Design review of the part built by this model. Coordinates are the model's own, in mm. Coordinates: 2 decimals unless noted, no trailing zeros. Write each loop counter-clockwise with the first axis right and the second up, starting at its lowest first coordinate (ties: lowest second). Pieces come first, ordered by that corner, then holes. Notation, with made-up numbers: (62.5, 66) - (113.5, 66) arc R18 cw to (113.5, 100) - close; hole circle Ø3 at (-29, 30). An arc over 180 degrees is marked (long way). Answer as CSV lines item,"result". Start each with the question number.
Q1. For line 1 along Z through (x, y) = (114.3, 1.85); line 2 along X through (y, z) = (3.7, 139.7); line 3 along X through (y, z) = (2.8, 117), list the stretches that pass through material, from the lowest coordinate up. Write a range as [from, to].
Q2. We need section A-A (z = 139.7). Write out the cut boundary in (x, y), plus the area to 3 significant figures.
Q3. We need section D-D (x = 12.7). Write out the cut boundary in (y, z).
Q4. We need section C-C (z = 38). Write out the cut boundary in (x, y).
Q5. Clearance check with flat-ended pins moving along their axes: pin 1 (2.5 mm diameter, centred on y = 3, z = 118.5, fed in from -X); pin 2 (1.4 mm diameter, centred on x = -6.5, y = 3.5, fed in from +Z). State where each tip first meets the part, or that it passes through.
Q6. We need section B-B (x = 114.3). Write out the cut boundary in (y, z), plus the area to 3 significant figures.
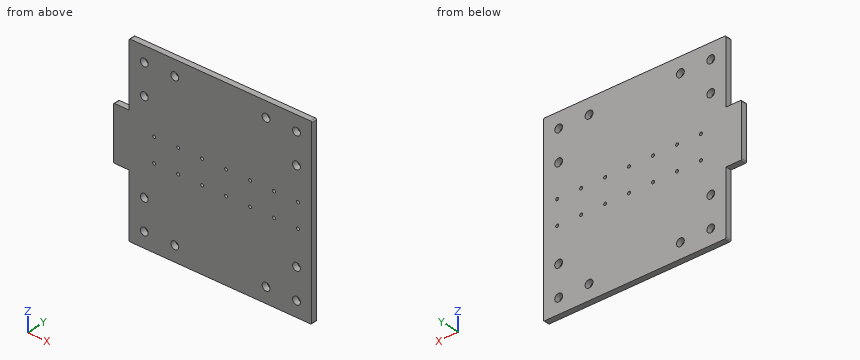
from build123d import *

# Parameters (mm, degrees)
SKETCH1_W             = 152.4
SKETCH1_H             = 152.4
SKETCH1_R             = 3.2639
SKETCH1_W_2           = 13.1
SKETCH1_H_2           = 45
BOSS_EXTRUDE1_DEPTH   = 4.7625
FILLET1_R             = 1
SKETCH11_R            = 1
CUT_EXTRUDE1_DEPTH    = 4.7625
M3X0_5_TAPPED_HOLE1_D = 2.5
LPATTERN1_COUNT       = 7
LPATTERN1_PITCH       = 20
LPATTERN1_COUNT_DIR2  = 2
LPATTERN1_PITCH_DIR2  = 20


with BuildPart() as part:
    # Sketch1 → Boss-Extrude1 (new body)
    # profile 1 of 2: a face of its own
    with BuildSketch(Plane(origin=(0, 0, 0), x_dir=(1, 0, 0), z_dir=(0, 1, 0))):
        with Locations((76.2, -76.2)):
            Rectangle(SKETCH1_W, SKETCH1_H)
        with Locations(Location((12.7, -12.7, 0), (0, 0, 90))):
            Circle(SKETCH1_R, mode=Mode.SUBTRACT)
        with Locations(Location((139.7, -12.7, 0), (0, 0, 90))):
            Circle(SKETCH1_R, mode=Mode.SUBTRACT)
        with Locations(Location((139.7, -139.7, 0), (0, 0, 90))):
            Circle(SKETCH1_R, mode=Mode.SUBTRACT)
        with Locations(Location((12.7, -139.7, 0), (0, 0, 90))):
            Circle(SKETCH1_R, mode=Mode.SUBTRACT)
        with Locations(Location((38.1, -12.7, 0), (0, 0, 90))):
            Circle(SKETCH1_R, mode=Mode.SUBTRACT)
        with Locations(Location((114.3, -12.7, 0), (0, 0, 90))):
            Circle(SKETCH1_R, mode=Mode.SUBTRACT)
        with Locations(Location((139.7, -38.1, 0), (0, 0, 90))):
            Circle(SKETCH1_R, mode=Mode.SUBTRACT)
        with Locations(Location((139.7, -114.3, 0), (0, 0, 90))):
            Circle(SKETCH1_R, mode=Mode.SUBTRACT)
        with Locations(Location((114.3, -139.7, 0), (0, 0, 90))):
            Circle(SKETCH1_R, mode=Mode.SUBTRACT)
        with Locations(Location((38.1, -139.7, 0), (0, 0, 90))):
            Circle(SKETCH1_R, mode=Mode.SUBTRACT)
        with Locations(Location((12.7, -114.3, 0), (0, 0, 90))):
            Circle(SKETCH1_R, mode=Mode.SUBTRACT)
        with Locations(Location((12.7, -38.1, 0), (0, 0, 90))):
            Circle(SKETCH1_R, mode=Mode.SUBTRACT)
    # profile 2 of 2: a face of its own
    with BuildSketch(Plane(origin=(0, 0, 0), x_dir=(1, 0, 0), z_dir=(0, 1, 0))):
        with Locations((-6.55, -76.2)):
            Rectangle(SKETCH1_W_2, SKETCH1_H_2)
    extrude(amount=BOSS_EXTRUDE1_DEPTH)

    # Fillet1
    fillet1_edges = [part.edges().sort_by_distance(p)[0] for p in [
        (152.4, 2.38125, 152.4),
        (0, 2.38125, 152.4),
        (-13.1, 2.38125, 98.7),
        (-13.1, 2.38125, 53.7),
        (0, 2.38125, 0),
        (152.4, 2.38125, 0),
    ]]
    fillet(fillet1_edges, radius=FILLET1_R)

    # Sketch11 → Cut-Extrude1 (cut)
    with BuildSketch(Plane(origin=(0, 4.7625, 0), x_dir=(1, 0, 0), z_dir=(0, 1, 0))):
        with Locations(Location((20.905, -87.2, 0), (0, 0, 270))):
            Circle(SKETCH11_R)
        with Locations(Location((20.905, -67.2, 0), (0, 0, 270))):
            Circle(SKETCH11_R)
        with Locations(Location((40.905, -87.2, 0), (0, 0, 270))):
            Circle(SKETCH11_R)
        with Locations(Location((40.905, -67.2, 0), (0, 0, 270))):
            Circle(SKETCH11_R)
        with Locations(Location((60.905, -87.2, 0), (0, 0, 270))):
            Circle(SKETCH11_R)
        with Locations(Location((60.905, -67.2, 0), (0, 0, 270))):
            Circle(SKETCH11_R)
        with Locations(Location((80.905, -87.2, 0), (0, 0, 270))):
            Circle(SKETCH11_R)
        with Locations(Location((80.905, -67.2, 0), (0, 0, 270))):
            Circle(SKETCH11_R)
        with Locations(Location((100.905, -87.2, 0), (0, 0, 270))):
            Circle(SKETCH11_R)
        with Locations(Location((100.905, -67.2, 0), (0, 0, 270))):
            Circle(SKETCH11_R)
        with Locations(Location((120.905, -87.2, 0), (0, 0, 270))):
            Circle(SKETCH11_R)
        with Locations(Location((120.905, -67.2, 0), (0, 0, 270))):
            Circle(SKETCH11_R)
        with Locations(Location((140.905, -87.2, 0), (0, 0, 270))):
            Circle(SKETCH11_R)
        with Locations(Location((140.905, -67.2, 0), (0, 0, 270))):
            Circle(SKETCH11_R)
    extrude(amount=-CUT_EXTRUDE1_DEPTH, mode=Mode.SUBTRACT)

    # M3x0.5 Tapped Hole1 (through all)
    with Locations(Plane(origin=(20.905, 4.7625, 67.2), x_dir=(0, 0, 1), z_dir=(0, 1, 0))):
        with Locations((0, 0)):
            m3x0_5_tapped_hole1 = Hole(M3X0_5_TAPPED_HOLE1_D / 2)

    # LPattern1: M3x0.5 Tapped Hole1 7 × 2
    with Locations(*[(i * LPATTERN1_PITCH, 0, j * LPATTERN1_PITCH_DIR2) for i in range(LPATTERN1_COUNT) for j in range(LPATTERN1_COUNT_DIR2) if (i, j) != (0, 0)]):
        add(m3x0_5_tapped_hole1, mode=Mode.SUBTRACT)


solid = part.part
Results list:
1,line 1,"z = [0, 9.44], [15.96, 136.44], [142.96, 152.4]"
1,line 2,"x = [0, 9.44], [15.96, 34.84], [41.36, 111.04], [117.56, 136.44], [142.96, 152.4]"
1,line 3,"x = [0, 10.87], [14.53, 137.87], [141.53, 152.4]"
2,outline,"(0, 0) - (9.44, 0) - (9.44, 4.76) - (0, 4.76) - close; (15.96, 0) - (34.84, 0) - (34.84, 4.76) - (15.96, 4.76) - close; (41.36, 0) - (111.04, 0) - (111.04, 4.76) - (41.36, 4.76) - close; (117.56, 0) - (136.44, 0) - (136.44, 4.76) - (117.56, 4.76) - close; (142.96, 0) - (152.4, 0) - (152.4, 4.76) - (142.96, 4.76) - close"
2,area,"601 mm2"
3,outline,"(0, 0) - (4.76, 0) - (4.76, 9.44) - (0, 9.44) - close; (0, 15.96) - (4.76, 15.96) - (4.76, 34.84) - (0, 34.84) - close; (0, 41.36) - (4.76, 41.36) - (4.76, 111.04) - (0, 111.04) - close; (0, 117.56) - (4.76, 117.56) - (4.76, 136.44) - (0, 136.44) - close; (0, 142.96) - (4.76, 142.96) - (4.76, 152.4) - (0, 152.4) - close"
4,outline,"(0, 0) - (9.44, 0) - (9.44, 4.76) - (0, 4.76) - close; (15.96, 0) - (136.44, 0) - (136.44, 4.76) - (15.96, 4.76) - close; (142.96, 0) - (152.4, 0) - (152.4, 4.76) - (142.96, 4.76) - close"
5,pin 1,"stops at x = 0"
5,pin 2,"stops at z = 98.7"
6,outline,"(0, 0) - (4.76, 0) - (4.76, 9.44) - (0, 9.44) - close; (0, 15.96) - (4.76, 15.96) - (4.76, 136.44) - (0, 136.44) - close; (0, 142.96) - (4.76, 142.96) - (4.76, 152.4) - (0, 152.4) - close"
6,area,"664 mm2"
